The model under review builds one solid part; all positions refer to its coordinate system, in mm. A direction names the side the tool comes from. Round coordinates to 2 decimals unless told otherwise and drop trailing zeros. Order: outer loops, then holes, each group sorted by start corner. A loop starts at its lowest first (then second) coordinate and runs counter-clockwise, first axis right, second up. Notation, with made-up numbers: M -5,20.5 L 1,20.5 A18 ccw 1,34.5 Z; hole C 75,24 d9. An arc over 180 degrees is marked long. Use a Markdown table: item, result. Add a question column.
1. Consider section B-B on y = -16.5. Count the separate pieces of the cut face and the enclosed holes in it, then the cut area to 3 significant figures.
2. Insertion check: P1, Ø12.5, axis at x = -206, y = -18.5, coming from the -Z side; P2, Ø1.5, axis at x = -100.5, z = 318.5, coming from the +Y side; P3, Ø2.5, axis at x = -66, z = -84.5, coming from the -Y side; P4, Ø2, axis at y = -3.5, z = 128.5, coming from the -X side. Each pin has a flat end and moves straight along its axis. Give the tip position at first contact, or say it passes through.
3. Consider section A-A on z = -25. State the section outline as (x, y) points.
4. The part is to be moulded in two halves that separate along Z. For faces 1 (the flat face through (12, -17, 97.869)), 2 (the flat face through (12, -17, 124.063)), 3 (the flat face through (12, -13, -253.35)), 4 (the flat face through (243.423, -13, 513)), say which applies: +Z half, -Z half, draft (parallel to the pull), parting line (faces both ways), or undercut.
5. To check wall thickness, follow probe 1 along X at (y, z) = (-2, 146). State the ranges of the line that lie inside material, in increasing order.
6. For faces 5 (the flat face through (18, -13, 538.401)), 6 (the flat face through (12, -17, 31.988)), 7 (the flat face through (218.023, -13, 112)), list the 3-axis set-ups (+Z, -Z, +X, -X, +Y, -Y) from which the entire face can be reached by the end or side of a thin tool; tool diameter is ignored.
from build123d import *

# Parameters (mm, degrees)
F1_DEPTH = 25.4
F2_W     = 406.4
F2_H     = 3.175
F3_DEPTH = 17.4625


# Not quite as in the source:
# - a feature names something its author has since deleted; it is built from what else it names


with BuildPart() as f1:
    # F0 (on Front) → F1 (new body)
    with BuildSketch(Plane.XZ):
        Polygon((218.0226445198, -253.3499094963), (218.0226445198, 487.6006533037), (243.4226445198, 487.6006533037), (243.4226445198, 538.4006533037), (-213.7773554802, 538.4006533037), (-213.7773554802, 487.6006533037), (-188.3773554802, 487.6006533037), (-188.3773554802, -253.3499094963), align=None)
    extrude(amount=F1_DEPTH)

    # F2 (on face) → F3 (cut)
    with BuildSketch(Plane.XZ.offset(25.4)):
        with Locations((14.8226445198, 168.5131533037)):
            Rectangle(F2_W, F2_H)
        with Locations((14.8226445198, 145.4944033037)):
            Rectangle(F2_W, F2_H)
        with Locations((14.8226445198, 122.4756533037)):
            Rectangle(F2_W, F2_H)
        with Locations((14.8226445198, 7.3819033037)):
            Rectangle(F2_W, F2_H)
        with Locations((14.8226445198, 76.4381533037)):
            Rectangle(F2_W, F2_H)
        with Locations((14.8226445198, 53.4194033037)):
            Rectangle(F2_W, F2_H)
        with Locations((14.8226445198, 99.4569033037)):
            Rectangle(F2_W, F2_H)
        with Locations((14.8226445198, 30.4006533037)):
            Rectangle(F2_W, F2_H)
        with Locations((14.8226445198, -15.6368466963)):
            Rectangle(F2_W, F2_H)
        with Locations((14.8226445198, -38.6555966963)):
            Rectangle(F2_W, F2_H)
        with Locations((14.8226445198, -61.6743466963)):
            Rectangle(F2_W, F2_H)
        with Locations((14.8226445198, -84.6930966963)):
            Rectangle(F2_W, F2_H)
        with Locations((14.8226445198, -107.7118466963)):
            Rectangle(F2_W, F2_H)
    extrude(amount=-F3_DEPTH, mode=Mode.SUBTRACT)


solid = f1.part
Answer block:
| question | item | result |
|---|---|---|
| 1 | separate pieces | 14 |
| 1 | enclosed holes | 0 |
| 1 | area | 308,000 mm^2 |
| 2 | P1 | z = 487.6 |
| 2 | P2 | y = 0 |
| 2 | P3 | y = -7.94 |
| 2 | P4 | x = -188.38 |
| 3 | outline | M -188.38,-25.4 L 218.02,-25.4 L 218.02,0 L -188.38,0 Z |
| 4 | face 1 | undercut |
| 4 | face 2 | undercut |
| 4 | face 3 | -Z half |
| 4 | face 4 | draft |
| 5 | probe 1 | -188.38 to 218.02 |
| 6 | face 5 | +Z, +X, -X, +Y, -Y |
| 6 | face 6 | +X, -X, -Y |
| 6 | face 7 | -Z, +X, +Y, -Y |
